```python
from build123d import *

# Parameters (mm, degrees)
F0_W      = 120.473326
F0_H      = 108.647734
F1_DEPTH  = 25
F3_R      = 5.08
F2_W      = 120.473326
F2_H      = 108.647734
F2_R      = 10.490665
F4_DEPTH  = 25.4
F4_FACE_W = 120.473326
F4_FACE_H = 108.647734
F4_FACE_R = 10.490665
F5_DEPTH  = 25.4


with BuildPart() as f1:
    # F0 (on Top) → F1 (new body)
    with BuildSketch(Plane.XY):
        Rectangle(F0_W, F0_H)
    extrude(amount=-F1_DEPTH)

    # F3
    f3_edges = [f1.edges().sort_by_distance(p)[0] for p in [
        (0, -54.323867, -25),
        (-60.236663, 0, -25),
        (0, 54.323867, -25),
        (60.236663, 0, -25),
        (60.236663, -54.323867, -12.5),
        (60.236663, 0, 0),
        (60.236663, 54.323867, -12.5),
        (-60.236663, -54.323867, -12.5),
        (0, -54.323867, 0),
        (-60.236663, 0, 0),
        (0, 54.323867, 0),
        (-60.236663, 54.323867, -12.5),
    ]]
    fillet(f3_edges, radius=F3_R)

    # F2 (on face) → F4 (join)
    with BuildSketch(Plane.XY):
        Rectangle(F2_W, F2_H)
        with Locations((-36.585487, -28.455362)):
            Circle(F2_R, mode=Mode.SUBTRACT)
        with Locations((36.585487, -28.455362)):
            Circle(F2_R, mode=Mode.SUBTRACT)
        with Locations((-36.585487, 28.455362)):
            Circle(F2_R, mode=Mode.SUBTRACT)
        with Locations((36.585487, 28.455362)):
            Circle(F2_R, mode=Mode.SUBTRACT)
    extrude(amount=-F4_DEPTH)

    # F4_face (on face) → F5 (join)
    with BuildSketch(Plane(origin=(0, 0, -25.4), x_dir=(1, 0, 0), z_dir=(0, 0, -1))):
        Rectangle(F4_FACE_W, F4_FACE_H)
        with Locations((-36.585487, 28.455362)):
            Circle(F4_FACE_R, mode=Mode.SUBTRACT)
        with Locations((36.585487, 28.455362)):
            Circle(F4_FACE_R, mode=Mode.SUBTRACT)
        with Locations((-36.585487, -28.455362)):
            Circle(F4_FACE_R, mode=Mode.SUBTRACT)
        with Locations((36.585487, -28.455362)):
            Circle(F4_FACE_R, mode=Mode.SUBTRACT)
    extrude(amount=F5_DEPTH)


solid = f1.part
```
Build history of the part. All positions in model axes, mm. A direction names the side the tool comes from. Round coordinates to 2 decimals unless told otherwise and drop trailing zeros. Loops run counter-clockwise (first coordinate to the right, second up) from the corner with the lowest first, then second, coordinate; pieces in that order, holes last.
Item 1: Pin check, flat tip, straight feed: P1, Ø17, axis at x = -36.59, y = -28.46, coming from the -Z side. Stop position of the tip, or through.
Item 2: Saw through at A-A (x = -40). List the corners of the cut face in (y, z), then the cut area to 3 significant figures.
Item 3: Drill centre lines: line 1 along Y through (x, z) = (36, -30); line 2 along Y through (x, z) = (-45, -47); line 3 along X through (y, z) = (36, -26). Where is each one in solid material? Low to high.
Item 4: Saw through at C-C (y = -25.5). List the corners of the cut face in (x, z), then the cut area to 3 significant figures.
Item 5: Saw through at B-B (z = -33). List the corners of the cut face in (x, y).
Item 6: Which spindle directions (+Z, -Z, +X, -X, +Y, -Y) get a long thin tool onto all of the face, cutting with end or side? Do faces 1 (the face through (-37, -28, -25)), 2 (the face through (-1, 1, 0)). Say none if no direction does.
Item 7: Two-plate mould, pull along Y, no slides. Class faces 3 (the face through (-1, -1, -50.8)), 4 (the face through (36, 29, -25)), 5 (the face through (-1, 54.324, -25)): released by +Y, released by -Y, zero draft, split by the parting line, or undercut.
Worked answers:
1. P1: stops at z = -25
2. outline: (-54.32, -50.8) - (-38.37, -50.8) - (-38.37, -25) - (-18.54, -25) - (-18.54, -50.8) - (18.54, -50.8) - (18.54, -25) - (38.37, -25) - (38.37, -50.8) - (54.32, -50.8) - (54.32, 0) - (-54.32, 0) - close
2. area: 4,500 mm2
3. line 1: y = -54.32 to -38.93, -17.98 to 17.98, 38.93 to 54.32
3. line 2: y = -54.32 to -34.72, -22.19 to 22.19, 34.72 to 54.32
3. line 3: x = -60.24 to -43.87, -29.3 to 29.3, 43.87 to 60.24
4. outline: (-60.24, -50.8) - (-46.65, -50.8) - (-46.65, -25) - (-26.52, -25) - (-26.52, -50.8) - (26.52, -50.8) - (26.52, -25) - (46.65, -25) - (46.65, -50.8) - (60.24, -50.8) - (60.24, 0) - (-60.24, 0) - close
4. area: 5,080 mm2
5. outline: (-60.24, -54.32) - (60.24, -54.32) - (60.24, 54.32) - (-60.24, 54.32) - close; hole circle Ø20.98 at (-36.59, -28.46); hole circle Ø20.98 at (-36.59, 28.46); hole circle Ø20.98 at (36.59, -28.46); hole circle Ø20.98 at (36.59, 28.46)
6. face 1: -Z
6. face 2: +Z, +X, -X, +Y, -Y
7. face 3: zero draft
7. face 4: undercut
7. face 5: released by +Y
